Check sheet for the modelled part. Datum: model origin and axes. Units: mm. A direction names the side the tool comes from. Round coordinates to 2 decimals unless told otherwise and drop trailing zeros. Loops run counter-clockwise (first coordinate to the right, second up) from the corner with the lowest first, then second, coordinate; pieces in that order, holes last. Notation, with made-up numbers: (-34, 62) -> (-3, 62) arc R15 cw to (-3, 84) -> close; hole circle Ø1 at (56.25, 21.5). An arc over 180 degrees is marked (long way). Use one line per item in the form item = value. Start each with the question number.
(1) Sectioned sample at B-B (y = -10.75). Record the cut outline in (x, z) (3 decimals), and give its area (3 significant figures).
(2) Draft check along Y on faces 3 (the cylindrical face through (5.22, -6.15, 0)), 4 (the flat face through (17, -8, 0.245)). Enter one of: released by +Y, released by -Y, zero draft, split by the parting line, or undercut.
(3) Material ranges on probe 1 along Y at (x, z) = (6.35, 0.05); probe 2 along Y at (x, z) = (32, 0.1); probe 3 along Y at (x, z) = (5, -0.1), recorded low to high. Write a range as [from, to].
(4) Set-up check for faces 1 (the cylindrical face through (6.67, -9.47, 0)), 2 (the cylindrical face through (27.553, -9.579, 0.003)): record each of +Z, -Z, +X, -X, +Y, -Y from which the full face is reachable in a straight line by a thin tool's end or side.
(5) Sectioned sample at C-C (z = -0.1). Record the cut outline in (x, y) (3 decimals), and give its area (3 significant figures).
(6) Sectioned sample at A-A (x = 6.35). Record the cut outline in (y, z) (3 decimals), and give its area (4 significant figures).
from build123d import *

# Parameters (mm, degrees)
SKETCH1_W             = 34.925
SKETCH1_H             = 15.84
BOSS_EXTRUDE1_DEPTH   = 0.245
CUT_EXTRUDE1_DEPTH    = 39.352331415
F_8_CLEARANCE_HOLE1_D = 4.9149


with BuildPart() as part:
    # Sketch1 → Boss-Extrude1 (new, symmetric)
    with BuildSketch(Plane.XY):
        with Locations((17.4625, -7.92)):
            Rectangle(SKETCH1_W, SKETCH1_H)
    extrude(amount=BOSS_EXTRUDE1_DEPTH, both=True)

    # Sketch2 → Cut-Extrude1 (cut, through all)
    with BuildSketch(Plane.XY.offset(0.245)):
        with BuildLine():
            Line((34.925, -5.88), (28.649421715, -5.88))
            ThreePointArc((28.649421715, -5.88), (27.564421715, -6.329421715), (27.115, -7.414421715))
            Line((27.115, -7.414421715), (27.115, -8.505578285))
            ThreePointArc((27.115, -8.505578285), (27.564421715, -9.590578285), (28.649421715, -10.04))
            Line((28.649421715, -10.04), (34.925, -10.04))
            Line((34.925, -10.04), (34.925, -5.88))
        make_face()
    extrude(amount=-CUT_EXTRUDE1_DEPTH, mode=Mode.SUBTRACT)

    # #8 Clearance Hole1 (through all)
    with Locations(Plane.XY.offset(0.245)):
        with Locations((6.35, -3.96875), (6.35, -11.90625)):
            Hole(F_8_CLEARANCE_HOLE1_D / 2)


solid = part.part
Checks:
q1.outline = (0, -0.245) -> (4.182, -0.245) -> (4.182, 0.245) -> (0, 0.245) -> close; (8.518, -0.245) -> (34.925, -0.245) -> (34.925, 0.245) -> (8.518, 0.245) -> close
q1.area = 15.0 mm2
q2.face_3 = undercut
q2.face_4 = zero draft
q3.probe_1 = [-15.84, -14.36], [-9.45, -6.43], [-1.51, 0]
q3.probe_2 = [-15.84, -10.04], [-5.88, 0]
q3.probe_3 = [-15.84, -13.96], [-9.85, -6.02], [-1.92, 0]
q4.face_1 = +Z, -Z
q4.face_2 = +Z, -Z, +X
q5.outline = (0, -15.84) -> (34.925, -15.84) -> (34.925, -10.04) -> (28.649, -10.04) arc R1.534 cw to (27.115, -8.506) -> (27.115, -7.414) arc R1.534 cw to (28.649, -5.88) -> (34.925, -5.88) -> (34.925, 0) -> (0, 0) -> close; hole circle Ø4.915 at (6.35, -11.906); hole circle Ø4.915 at (6.35, -3.969)
q5.area = 484 mm2
q6.outline = (-15.84, -0.245) -> (-14.364, -0.245) -> (-14.364, 0.245) -> (-15.84, 0.245) -> close; (-9.449, -0.245) -> (-6.426, -0.245) -> (-6.426, 0.245) -> (-9.449, 0.245) -> close; (-1.511, -0.245) -> (0, -0.245) -> (0, 0.245) -> (-1.511, 0.245) -> close
q6.area = 2.945 mm2
